Job drawing, mm, ordinate dimensions from the low corner. One solid piece. A direction names the side the tool comes from. Coordinates: 2 decimals unless noted, no trailing zeros. Order: outer loops, then holes, each group sorted by start corner. A loop starts at its lowest first (then second) coordinate and runs counter-clockwise, first axis right, second up. Notation, with made-up numbers: (59, 2) -> (82, 2) arc R11 cw to (82, 16) -> close; hole circle Ø2 at (61, 17). An arc over 180 degrees is marked (long way). Use CSV: the item, a comma, the result in double quotes. Start each with the question number.
(1) Cut at A-A on z = 1.7. Write the cut outline in (x, y), plus the area to 4 significant figures.
(2) Probe L1, parallel to X at y = 16.25, z = 2.2; L2, parallel to Y at x = 23.25, z = 2.5. List the from-to ranges inside material, lowest first.
(3) Pull direction Z, two halves, no side cores. Call the marked faces 1, 2 and 3: pulls with the +Z half, pulls with the -Z half, needs draft (parallel to the pull), parting line crosses it, or undercut.
(4) Tool access for the marked faces 4, 5, 6 and 7: list every direction of +Z, -Z, +X, -X, +Y, -Y with a clear straight run to the whole face (end or side of a thin tool).
(5) Cut at C-C on y = 16.75. Write the cut outline in (x, z).
(6) Cut at B-B on x = 22.25. Write the cut outline in (y, z), plus the area to 3 significant figures.
(7) Pin check, flat tips, straight feed: pin 1 Ø1.6 at (y, z) = (1, 2.5) entering from +X; pin 2 Ø1 at (x, z) = (1, 2.5) entering from +Y; pin 3 Ø1 at (x, z) = (1.5, 2) entering from -Y. Stop position of each tip, or through.
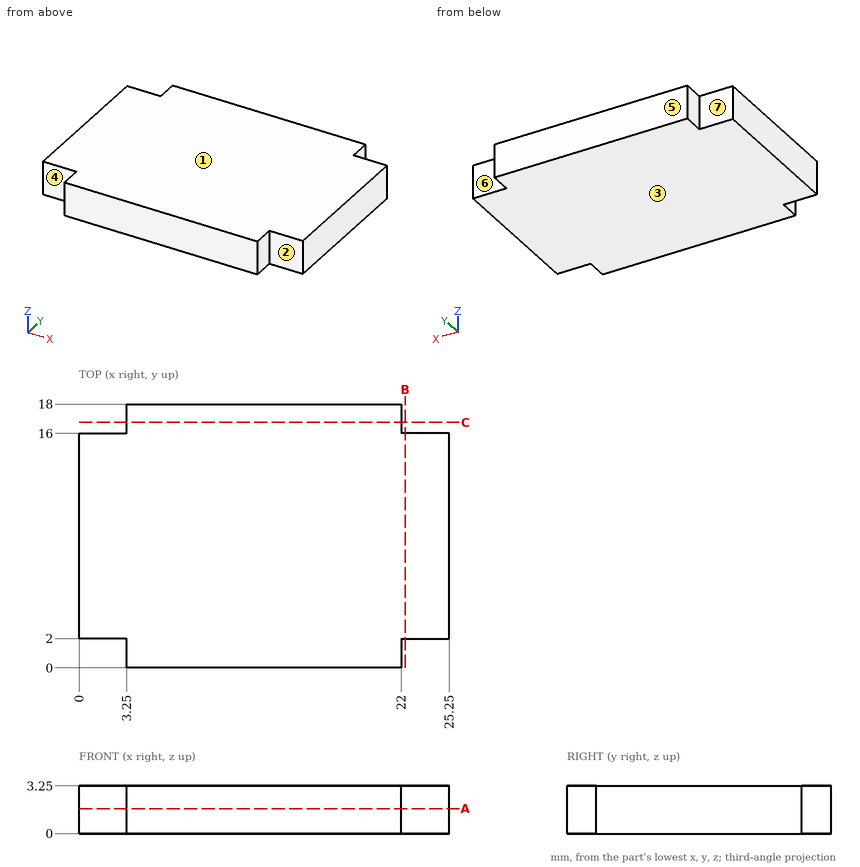
Outcome:
1,outline,"(0, 2) -> (3.25, 2) -> (3.25, 0) -> (22, 0) -> (22, 2) -> (25.25, 2) -> (25.25, 16) -> (22, 16) -> (22, 18) -> (3.25, 18) -> (3.25, 16) -> (0, 16) -> close"
1,area,"428.5 mm2"
2,L1,"3.25 to 22"
2,L2,"2 to 16"
3,face 1,"pulls with the +Z half"
3,face 2,"needs draft"
3,face 3,"pulls with the -Z half"
4,face 4,"+Z, -Z, -X, -Y"
4,face 5,"+Z, -Z, +X, -X, +Y"
4,face 6,"+Z, -Z, +X, +Y"
4,face 7,"+Z, -Z, -X, +Y"
5,outline,"(3.25, 0) -> (22, 0) -> (22, 3.25) -> (3.25, 3.25) -> close"
6,outline,"(2, 0) -> (16, 0) -> (16, 3.25) -> (2, 3.25) -> close"
6,area,"45.5 mm2"
7,pin 1,"x = 22"
7,pin 2,"y = 16"
7,pin 3,"y = 2"
